The listing builds one solid part. Answer for the finished solid, in the listing's coordinates (mm). A direction names the side the tool comes from. Coordinates: 2 decimals unless noted, no trailing zeros. Order: outer loops, then holes, each group sorted by start corner. A loop starts at its lowest first (then second) coordinate and runs counter-clockwise, first axis right, second up. Notation, with made-up numbers: (-12, -23) -> (47, -23) arc R18 ccw to (47, -5) -> close; hole circle Ø9 at (79.5, -23). An arc over 180 degrees is marked (long way). Answer in a Markdown table with one row per item.
```python
from build123d import *

# Parameters (mm, degrees)
F2_DEPTH = 5
F4_DEPTH = 120
F6_DEPTH = 118


with BuildPart() as f2:
    # F0 (on Front) → F2 (new body)
    with BuildSketch(Plane.XZ):
        Polygon((40.23458, -40.23458), (56.900289, 0), (40.23458, 40.23458), (0, 56.900289), (-40.23458, 40.23458), (-56.900289, 0), (-40.23458, -40.23458), (0, -56.900289), align=None)
    extrude(amount=F2_DEPTH)

    # F3 (on offset) → F4 (join)
    with BuildSketch(Plane.XZ.offset(5)):
        Polygon((37.659568, -37.659568), (53.258672, 0), (37.659568, 37.659568), (0, 53.258672), (-37.659568, 37.659568), (-53.258672, 0), (-37.659568, -37.659568), (0, -53.258672), align=None)
    extrude(amount=F4_DEPTH)

    # F5 (on face) → F6 (cut)
    with BuildSketch(Plane.XZ.offset(125)):
        Polygon((35.406429, -35.406429), (50.072253, 0), (35.406429, 35.406429), (0, 50.072253), (-35.406429, 35.406429), (-50.072253, 0), (-35.406429, -35.406429), (0, -50.072253), align=None)
    extrude(amount=-F6_DEPTH, mode=Mode.SUBTRACT)


solid = f2.part
```
(1) Find the intervals of material crossed by line 1 along Y through (x, z) = (-6, -26); line 2 along Y through (x, z) = (13.5, -50.5); line 3 along Z through (x, y) = (6, -69), in increasing order. Write a range as from..to.
Check values:
| item | result |
|---|---|
| line 1 | -7..0 |
| line 2 | -5..0 |
| line 3 | -50.77..-47.59, 47.59..50.77 |
(2) Which of the six approach directions +Z, -Z, +X, -X, +Y, -Y give full straight-line access (tool end or side, diameter ignored) to faces 5 (the flat face through (45.35, -64.16, -19.09)), 6 (the flat face through (19.09, -64.16, 45.35)), 7 (the flat face through (-45.568, -64.16, -18.566)), 8 (the flat face through (46, -5, -21))?
Check values:
| item | result |
|---|---|
| face 5 | -Z, +X, -Y |
| face 6 | +Z, +X, -Y |
| face 7 | -Z, -X, -Y |
| face 8 | -Y |
(3) A cutting plane is placed at A-A, the plane y = -37.5. Determine the outline of the cut face in (x, z).
Check values:
| item | result |
|---|---|
| outline | (-53.26, 0) -> (-37.66, -37.66) -> (0, -53.26) -> (37.66, -37.66) -> (53.26, 0) -> (37.66, 37.66) -> (0, 53.26) -> (-37.66, 37.66) -> close; hole (-50.07, 0) -> (-35.41, -35.41) -> (0, -50.07) -> (35.41, -35.41) -> (50.07, 0) -> (35.41, 35.41) -> (0, 50.07) -> (-35.41, 35.41) -> close |
(4) A cutting plane is placed at C-C, the plane x = -44. Determine the outline of the cut face in (y, z).
Check values:
| item | result |
|---|---|
| outline | (-125, -22.35) -> (-5, -22.35) -> (-5, -31.14) -> (0, -31.14) -> (0, 31.14) -> (-5, 31.14) -> (-5, 22.35) -> (-125, 22.35) -> (-125, 14.66) -> (-7, 14.66) -> (-7, -14.66) -> (-125, -14.66) -> close |
(5) For a pull along Z with two mould halves and no side action, classify faces 1 (the flat face through (-1, 0, 1)), 2 (the flat face through (48.45, -2.46, -20.4)), 3 (the flat face through (-17.951, -66.826, -42.637)), 4 (the flat face through (-18.566, -64.16, 45.568)) as released by +Z, released by -Z, zero draft, split by the parting line, or undercut.
Check values:
| item | result |
|---|---|
| face 1 | zero draft |
| face 2 | released by -Z |
| face 3 | undercut |
| face 4 | released by +Z |
(6) Flat-ended cylindrical pins translate along their axes: pin 1 (5 mm diameter, centred on y = -99.5, z = 2, fed in from +X); pin 2 (1.5 mm diameter, centred on x = -41, y = -59.5, fed in from -Z); pin 3 (8 mm diameter, centred on y = -18, z = 30, fed in from -X). Find the tip coordinate at first contact, or state that the pin passes through.
Check values:
| item | result |
|---|---|
| pin 1 | x = 53.26 |
| pin 2 | z = -31.41 |
| pin 3 | x = -42.49 |
(7) A cutting plane is placed at B-B, the plane z = 30. Determine the outline of the cut face in (x, y).
Check values:
| item | result |
|---|---|
| outline | (-44.47, -5) -> (-40.83, -5) -> (-40.83, -125) -> (-37.65, -125) -> (-37.65, -7) -> (37.65, -7) -> (37.65, -125) -> (40.83, -125) -> (40.83, -5) -> (44.47, -5) -> (44.47, 0) -> (-44.47, 0) -> close |
